Input: part model. Units: mm. Frame: model coordinates. Face numbers are marked on the shaded views. A direction names the side the tool comes from. Give positions to 0.01 mm unless a question says otherwise; leave off trailing zeros. Order: outer loops, then holes, each group sorted by start corner. A loop starts at its lowest first (then second) coordinate and runs counter-clockwise, first axis right, second up. Notation, with made-up numbers: (85.5, 43) - (137.5, 43) arc R27 ccw to (137.5, 61) - close; hole circle Ø7 at (20.5, 13.5). An arc over 180 degrees is marked (long way). Answer in a Markdown table with one row per item. Add a question column.
1. Contact query for flat-ended pins moving along their axis: pin 1 (4 mm diameter, centred on y = 9.5, z = 3.5, fed in from +X); pin 2 (1 mm diameter, centred on x = 2, z = -7, fed in from +Y); pin 3 (1 mm diameter, centred on y = 6, z = 2.5, fed in from -X). Output: stop coordinate, or through.
2. Section query B-B on z = 0.5. Count the separate pieces of the cut face and the enclosed holes in it, and give its area (3 significant figures).
3. Access query for the marked faces 5, 6 and 7. Directions: +Z, -Z, +X, -X, +Y, -Y. A direction counts if a zero-diameter tool reaches every point of the face in a straight line with its end or side. Return the directions, or none.
4. Section query C-C on y = 6.25. Return loops of the section in (x, z), and give its area (3 significant figures).
5. Ray query, line 1 (X direction, y = 13, z = 6.5); line 2 (X direction, y = 7, z = 2.25); line 3 (Y direction, x = 5.6, z = 0.5). Return the intervals inside material, ascending. Write a range as [from, to].
6. Mould query, pull axis Z, two halves, no side actions, for the marked faces 1, 2, 3 and 4. Classes: released by +Z, released by -Z, zero draft, split by the parting line, or undercut.
```python
from build123d import *

# Parameters (mm, degrees)
SKETCH2_R               = 7.5
SKETCH3_R               = 8.5
SKETCH9_W               = 8.5
SKETCH9_H               = 24.609106297
CUT_EXTRUDE1_DEPTH      = 10
CUT_EXTRUDE1_DEPTH_BACK = 10
CUT_EXTRUDE2_DEPTH      = 10
CUT_EXTRUDE2_DEPTH_BACK = 10
CUT_EXTRUDE3_DEPTH      = 14
FILLET1_R               = 1
SKETCH12_R              = 1.25
CUT_EXTRUDE4_DEPTH      = 30


with BuildPart() as part:
    # Sketch2 → Loft1 section 0
    with BuildSketch(Plane(origin=(0, 22, 0), x_dir=(1, 0, 0), z_dir=(0, 1, 0))):
        Circle(SKETCH2_R)
    # Sketch3 → Loft1 section 1
    with BuildSketch(Plane(origin=(0, 0, 0), x_dir=(1, 0, 0), z_dir=(0, 1, 0))):
        Circle(SKETCH3_R)
    loft()

    # Sketch9 → Cut-Extrude1 (cut, two sides)
    with BuildSketch(Plane.XY) as cut_extrude1_sk:
        with Locations((0, 23.304553149)):
            Rectangle(SKETCH9_W, SKETCH9_H)
    extrude(amount=CUT_EXTRUDE1_DEPTH, mode=Mode.SUBTRACT)
    extrude(cut_extrude1_sk.sketch, amount=-CUT_EXTRUDE1_DEPTH_BACK, mode=Mode.SUBTRACT)

    # Sketch10 → Cut-Extrude2 (cut, two sides)
    with BuildSketch(Plane(origin=(0, 0, 0), x_dir=(0, 0, -1), z_dir=(1, 0, 0))) as cut_extrude2_sk:
        with BuildLine():
            ThreePointArc((1.551397817, 22.278129211), (-3.230375863, 20.336914385), (-6.681717999, 16.5))
            Line((-6.681717999, 16.5), (-6.777720856, 11))
            Line((-6.777720856, 11), (-14.541953313, 11))
            Line((-14.541953313, 11), (-14.541953313, 25.761445422))
            Line((-14.541953313, 25.761445422), (14.965624753, 25.761445422))
            Line((14.965624753, 25.761445422), (14.965624753, 11))
            Line((14.965624753, 11), (6.777720856, 11))
            Line((6.777720856, 11), (6.043769414, 23))
            Line((6.043769414, 23), (1.551397817, 22.278129211))
        make_face()
    extrude(amount=CUT_EXTRUDE2_DEPTH, mode=Mode.SUBTRACT)
    extrude(cut_extrude2_sk.sketch, amount=-CUT_EXTRUDE2_DEPTH_BACK, mode=Mode.SUBTRACT)

    # Sketch11 → Cut-Extrude3 (cut)
    with BuildSketch(Plane(origin=(0, 0, 0), x_dir=(-1, 0, 0), z_dir=(0, -1, 0))):
        with BuildLine():
            Line((4.25, -4.5), (4.25, 4.5))
            ThreePointArc((4.25, 4.5), (0, 5.448066505), (-4.25, 4.5))
            Line((-4.25, 4.5), (-4.25, -4.5))
            ThreePointArc((-4.25, -4.5), (0, -5.448066505), (4.25, -4.5))
        make_face()
    extrude(amount=-CUT_EXTRUDE3_DEPTH, mode=Mode.SUBTRACT)

    # Fillet1
    fillet1_edges = [part.edges().sort_by_distance(p)[0] for p in [
        (4.303290893, 22, -6.104932034),
        (-4.303290893, 22, -6.104932034),
    ]]
    fillet(fillet1_edges, radius=FILLET1_R)

    # Sketch12 → Cut-Extrude4 (cut, symmetric)
    with BuildSketch(Plane(origin=(0, 0, 0), x_dir=(0, 0, -1), z_dir=(1, 0, 0))):
        with Locations((-0.5, 15.25)):
            Circle(SKETCH12_R)
    extrude(amount=CUT_EXTRUDE4_DEPTH, both=True, mode=Mode.SUBTRACT)


solid = part.part
```
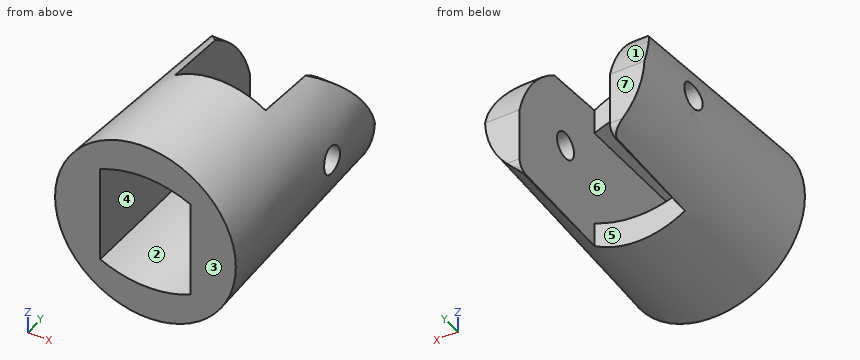
Answer:
| question | item | result |
|---|---|---|
| 1 | pin 1 | stops at x = 7.94 |
| 1 | pin 2 | stops at y = 11 |
| 1 | pin 3 | stops at x = -7.98 |
| 2 | separate pieces | 4 |
| 2 | enclosed holes | 0 |
| 2 | area | 145 mm² |
| 3 | face 5 | +Z, -Z, +Y |
| 3 | face 6 | +Y |
| 3 | face 7 | +Z, -Z, +X, -X, +Y |
| 4 | outline | circle Ø16.43 at (0, 0); hole (-4.25, -4.5) arc R10 ccw to (4.25, -4.5) - (4.25, 4.5) arc R10 ccw to (-4.25, 4.5) - close |
| 4 | area | 125 mm² |
| 5 | line 1 | x = [-4.51, -4.25], [4.25, 4.51] |
| 5 | line 2 | x = [-7.87, -4.25], [4.25, 7.87] |
| 5 | line 3 | y = [0, 14], [16.5, 21.75] |
| 6 | face 1 | released by +Z |
| 6 | face 2 | undercut |
| 6 | face 3 | zero draft |
| 6 | face 4 | undercut |
